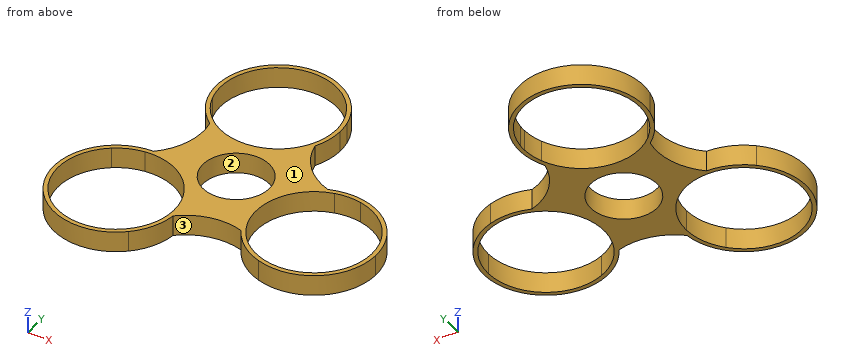
from build123d import *

# Parameters (mm, degrees)
F0_R     = 8
F1_DEPTH = 5


# Not quite as in the source:
# - a feature names something its author has since deleted; it is built from what else it names


with BuildPart() as f1:
    # F0 (on Top) → F1 (new body)
    with BuildSketch(Plane.XY):
        with BuildLine():
            ThreePointArc((7.9121440123, 17.5499293192), (9.1490120469, 20.8777196251), (9.5691464087, 24.4029881218))
            ThreePointArc((9.5691464087, 24.4029881218), (9.4793257017, 26.042059033), (9.2109392818, 27.6615002765))
            ThreePointArc((9.2109392818, 27.6615002765), (8.8193827537, 26.8385345747), (8.4785274274, 25.9933087425))
            ThreePointArc((8.4785274274, 25.9933087425), (8.5464733038, 25.1994382891), (8.5691464087, 24.4029881218))
            ThreePointArc((8.5691464087, 24.4029881218), (8.3311107472, 21.8323194251), (7.6250981876, 19.3490665605))
            ThreePointArc((7.6250981876, 19.3490665605), (7.7412805882, 18.4451358603), (7.9121440123, 17.5499293192))
        make_face()
        with BuildLine():
            ThreePointArc((8.4785274274, 25.9933087425), (8.8193827537, 26.8385345747), (9.2109392818, 27.6615002765))
            ThreePointArc((9.2109392818, 27.6615002765), (-8.689365746, 39.0447809948), (-20.0726464643, 21.144475967))
            ThreePointArc((-20.0726464643, 21.144475967), (-19.3800207125, 20.593183388), (-18.7211221359, 20.0019925512))
            ThreePointArc((-18.7211221359, 20.0019925512), (-8.442463209, 38.0752303486), (8.4785274274, 25.9933087425))
        make_face()
        with BuildLine():
            ThreePointArc((18.2808163885, 6.4299700246), (11.5832094425, 10.578918544), (7.9121440123, 17.5499293192))
            ThreePointArc((7.9121440123, 17.5499293192), (-2.0581580843, 9.7870747046), (-14.4218573571, 12.3962462122))
            ThreePointArc((-14.4218573571, 12.3962462122), (-14.7542295678, 4.6387919255), (-18.9207994891, -1.9131744502))
            ThreePointArc((-18.9207994891, -1.9131744502), (-7.9907957387, -6.1219111722), (-3.4181808461, -16.9047512351))
            ThreePointArc((-3.4181808461, -16.9047512351), (-3.4376551817, -17.6688525497), (-3.4960276219, -18.4309698155))
            ThreePointArc((-3.4960276219, -18.4309698155), (3.2731601147, -14.8661881946), (10.919943616, -15.1034068738))
            ThreePointArc((10.919943616, -15.1034068738), (9.655402449, -2.646349524), (18.2808163885, 6.4299700246))
        make_face()
        Circle(F0_R, mode=Mode.SUBTRACT)
        with BuildLine():
            ThreePointArc((-14.4218573571, 12.3962462122), (-2.0581580843, 9.7870747046), (7.9121440123, 17.5499293192))
            ThreePointArc((7.9121440123, 17.5499293192), (7.7412805882, 18.4451358603), (7.6250981876, 19.3490665605))
            ThreePointArc((7.6250981876, 19.3490665605), (-2.2534030631, 10.7683334455), (-14.907533277, 14.0980115505))
            ThreePointArc((-14.907533277, 14.0980115505), (-14.6395764677, 13.2542976843), (-14.4218573571, 12.3962462122))
        make_face()
        with BuildLine():
            ThreePointArc((-18.7211221359, 20.0019925512), (-19.3800207125, 20.593183388), (-20.0726464643, 21.144475967))
            ThreePointArc((-20.0726464643, 21.144475967), (-18.0308595518, 16.2642013697), (-14.4218573571, 12.3962462122))
            ThreePointArc((-14.4218573571, 12.3962462122), (-14.6395764677, 13.2542976843), (-14.907533277, 14.0980115505))
            ThreePointArc((-14.907533277, 14.0980115505), (-17.1908591544, 16.8067871532), (-18.7211221359, 20.0019925512))
        make_face()
        with BuildLine():
            ThreePointArc((20.1455918313, 6.0030413071), (19.2063911412, 6.1867474035), (18.2808163885, 6.4299700246))
            ThreePointArc((18.2808163885, 6.4299700246), (9.655402449, -2.646349524), (10.919943616, -15.1034068738))
            ThreePointArc((10.919943616, -15.1034068738), (11.7048264649, -15.3603839917), (12.474376183, -15.6601698438))
            ThreePointArc((12.474376183, -15.6601698438), (10.6520286886, -2.8250110982), (20.1455918313, 6.0030413071))
        make_face()
        with BuildLine():
            ThreePointArc((28.1221549341, 6.8802345627), (23.1634660922, 7.4860881247), (18.2808163885, 6.4299700246))
            ThreePointArc((18.2808163885, 6.4299700246), (19.2063911412, 6.1867474035), (20.1455918313, 6.0030413071))
            ThreePointArc((20.1455918313, 6.0030413071), (23.2091706485, 6.4871331239), (26.3041545683, 6.2848101329))
            ThreePointArc((26.3041545683, 6.2848101329), (27.2226565904, 6.5535105265), (28.1221549341, 6.8802345627))
        make_face()
        with BuildLine():
            ThreePointArc((-20.2929169032, -3.0308417387), (-19.5903609061, -2.4922611868), (-18.9207994891, -1.9131744502))
            ThreePointArc((-18.9207994891, -1.9131744502), (-24.0938941246, -3.0200013713), (-28.5610315871, -5.8538427275))
            ThreePointArc((-28.5610315871, -5.8538427275), (-27.6775469435, -5.7980858959), (-26.7988899679, -5.6903090014))
            ThreePointArc((-26.7988899679, -5.6903090014), (-23.7155132394, -3.9456513623), (-20.2929169032, -3.0308417387))
        make_face()
        with BuildLine():
            ThreePointArc((-3.4181808461, -16.9047512351), (-7.9907957387, -6.1219111722), (-18.9207994891, -1.9131744502))
            ThreePointArc((-18.9207994891, -1.9131744502), (-19.5903609061, -2.4922611868), (-20.2929169032, -3.0308417387))
            ThreePointArc((-20.2929169032, -3.0308417387), (-9.2053176863, -6.3632545482), (-4.4181808461, -16.9047512351))
            ThreePointArc((-4.4181808461, -16.9047512351), (-4.4869248616, -18.2904303809), (-4.6924818025, -19.6625013626))
            ThreePointArc((-4.6924818025, -19.6625013626), (-4.1118905803, -19.0296020384), (-3.4960276219, -18.4309698155))
            ThreePointArc((-3.4960276219, -18.4309698155), (-3.4376551817, -17.6688525497), (-3.4181808461, -16.9047512351))
        make_face()
        with BuildLine():
            ThreePointArc((38.8490344373, -7.4982368866), (35.8718628785, 1.471244496), (28.1221549341, 6.8802345627))
            ThreePointArc((28.1221549341, 6.8802345627), (27.2226565904, 6.5535105265), (26.3041545683, 6.2848101329))
            ThreePointArc((26.3041545683, 6.2848101329), (34.5815011117, 1.4914326892), (37.8490344373, -7.4982368866))
            ThreePointArc((37.8490344373, -7.4982368866), (31.7032518121, -19.0875107823), (18.6617102331, -20.5017620856))
            ThreePointArc((18.6617102331, -20.5017620856), (19.1377449469, -21.1766467253), (19.5759139405, -21.876708336))
            ThreePointArc((19.5759139405, -21.876708336), (32.81851582, -19.5210653278), (38.8490344373, -7.4982368866))
        make_face()
        with BuildLine():
            ThreePointArc((12.474376183, -15.6601698438), (11.7048264649, -15.3603839917), (10.919943616, -15.1034068738))
            ThreePointArc((10.919943616, -15.1034068738), (14.6052028869, -19.311431978), (19.5759139405, -21.876708336))
            ThreePointArc((19.5759139405, -21.876708336), (19.1377449469, -21.1766467253), (18.6617102331, -20.5017620856))
            ThreePointArc((18.6617102331, -20.5017620856), (15.2214583236, -18.5238856386), (12.474376183, -15.6601698438))
        make_face()
        with BuildLine():
            ThreePointArc((-26.7988899679, -5.6903090014), (-27.6775469435, -5.7980858959), (-28.5610315871, -5.8538427275))
            ThreePointArc((-28.5610315871, -5.8538427275), (-29.4690893537, -27.0476019762), (-8.275330105, -27.9556597428))
            ThreePointArc((-8.275330105, -27.9556597428), (-8.1635176407, -27.1041048739), (-8.003150447, -26.2603453792))
            ThreePointArc((-8.003150447, -26.2603453792), (-28.7533738733, -26.348467934), (-26.7988899679, -5.6903090014))
        make_face()
        with BuildLine():
            ThreePointArc((-8.275330105, -27.9556597428), (-5.0113342557, -23.6320437442), (-3.4960276219, -18.4309698155))
            ThreePointArc((-3.4960276219, -18.4309698155), (-4.1118905803, -19.0296020384), (-4.6924818025, -19.6625013626))
            ThreePointArc((-4.6924818025, -19.6625013626), (-5.9051240284, -23.183557577), (-8.003150447, -26.2603453792))
            ThreePointArc((-8.003150447, -26.2603453792), (-8.1635176407, -27.1041048739), (-8.275330105, -27.9556597428))
        make_face()
    extrude(amount=F1_DEPTH)


solid = f1.part
Could you check a few things on this model? Use its own coordinates, in mm. Face numbers are marked on the shaded views. Give positions to 0.01 mm unless a question says otherwise; leave off trailing zeros. Order: outer loops, then holes, each group sorted by start corner. A loop starts at its lowest first (then second) coordinate and runs counter-clockwise, first axis right, second up. Notation, with made-up numbers: M 87.5,69.5 L 134.5,69.5 A33 ccw 134.5,101.5 Z; hole C -16.75,37 d3. An arc over 180 degrees is marked long. One line per question, with ' | ' between items.
1. I want a section at B-B (y = 2). List the corners of the cut face in (x, z) for me.
Results:
outline: M -15.87,0 L -7.75,0 L -7.75,5 L -15.87,5 Z; M 7.75,0 L 13.56,0 L 13.56,5 L 7.75,5 Z; M 34.13,0 L 35.46,0 L 35.46,5 L 34.13,5 Z
2. I want a section at C-C (x = -6). List the corners of the cut face in (y, z) for me, and give its area (3 significant figures).
Results:
outline: M -25.32,0 L -23.37,0 L -23.37,5 L -25.32,5 Z; M -10.44,0 L -5.29,0 L -5.29,5 L -10.44,5 Z; M 5.29,0 L 10.41,0 L 10.41,5 L 5.29,5 Z; M 38.39,0 L 39.39,0 L 39.39,5 L 38.39,5 Z | area: 66.1 mm²
3. I want a section at D-D (x = 14). List the corners of the cut face in (y, z) for me.
Results:
outline: M -18.81,0 L -17.45,0 L -17.45,5 L -18.81,5 Z; M 2.45,0 L 8.49,0 L 8.49,5 L 2.45,5 Z
4. We'd pull the mould along Y, two halves only. Please class the marked faces 1, 2 and 3: +Y half, -Y half, draft (parallel to the pull), parting line (faces both ways), or undercut.
Results:
face 1: draft | face 2: undercut | face 3: -Y half
5. I'm going to push a flat-ended pin straight in: pin 1 (3 mm diameter, centred on y = 18.5, z = 4, fed in from -X). Where does the tip first touch, or does it pass through?
Results:
pin 1: x = -19.77
6. If I drill on line 1 (Y direction, x = 5.5, z = 0.45); line 2 (Y direction, x = 1.5, z = 1.3); line 3 (Y direction, x = -6, z = 3.25), over which ranges is the centre line in solid material (lowest first)?
Results:
line 1: -14.53 to -5.81, 5.81 to 15.66, 33.15 to 34.68 | line 2: -15.39 to -7.86, 7.86 to 12.24, 36.57 to 37.71 | line 3: -25.32 to -23.37, -10.44 to -5.29, 5.29 to 10.41, 38.39 to 39.39
7. I want a section at A-A (z = 1.7). List the corners of the cut face in (x, y) for me.
Results:
outline: M -18.92,-1.91 A15 ccw long -3.5,-18.43 A15 cw 10.92,-15.1 A15 ccw long 18.28,6.43 A15 cw 7.91,17.55 A15 ccw long -14.42,12.4 A15 cw Z; hole C -18.42,-16.9 d28; hole C -5.43,24.4 d28; hole C 0,0 d16; hole C 23.85,-7.5 d28
